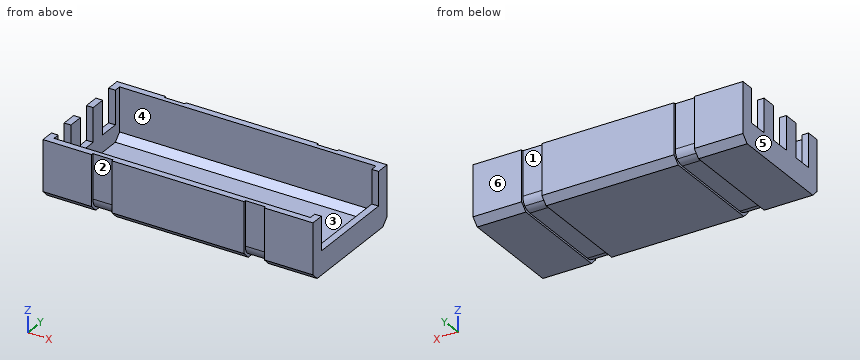
```python
from build123d import *

# Parameters (mm, degrees)
F0_W         = 40
F0_H         = 17.5
F1_DEPTH     = 8.5
F2_T         = -1
F3_W         = 1
F3_H         = 3
F4_DEPTH     = 5
F5_SIZE      = 1
F8_W         = 3
F8_H         = 1
F8_H_2       = 7.5
F11_DEPTH    = 0.3
F7_W         = 3
F7_H         = 1.4142135624
F12_DEPTH    = 0.3
F6_W         = 3
F6_H         = 15.5
F13_DEPTH    = 0.3
F9_W         = 3
F9_H         = 7.5
F14_DEPTH    = 0.3
F10_W        = 3
F10_H        = 5.3033008589
F10_H_2      = 1.4142135624
F15_DEPTH    = 0.3
F16_T1_DEPTH = 3
F16_T3_DEPTH = 3
F18_W        = 2.25
F18_H        = 5
F19_DEPTH    = 25


# Not quite as in the source:
# - a fillet or chamfer that OpenCascade refuses, or shapes differently, is made with other operations: its cross-section is extruded or revolved along the edge and cut away or added
# - two fillets or chamfers of one size are made in one step


with BuildPart() as f1:
    # F0 (on Top) → F1 (new body)
    with BuildSketch(Plane.XY):
        with Locations((-65.668810606, 16.5984117985)):
            Rectangle(F0_W, F0_H)
    extrude(amount=F1_DEPTH)

    # F2
    f2_openings = [f1.faces().sort_by_distance(p)[0] for p in [
        (-65.668811, 16.598412, 8.5),
    ]]
    offset(amount=F2_T, openings=f2_openings)

    # F3 (on face) → F4 (cut)
    with BuildSketch(Plane.XY.offset(8.5)):
        with Locations((-85.168810606, 21.8484117985)):
            Rectangle(F3_W, F3_H)
        with Locations((-85.168810606, 16.5984117985)):
            Rectangle(F3_W, F3_H)
        with Locations((-85.168810606, 11.3484117985)):
            Rectangle(F3_W, F3_H)
        with Locations((-46.168810606, 11.3484117985)):
            Rectangle(F3_W, F3_H)
        with Locations((-46.168810606, 16.5984117985)):
            Rectangle(F3_W, F3_H)
        with Locations((-46.168810606, 21.8484117985)):
            Rectangle(F3_W, F3_H)
    extrude(amount=-F4_DEPTH, mode=Mode.SUBTRACT)

    # F5
    f5_edges = [f1.edges().sort_by_distance(p)[0] for p in [
        (-65.668811, 7.848412, 0),
        (-65.668811, 25.348412, 0),
        (-65.668811, 24.348412, 1),
        (-65.668811, 8.848412, 1),
    ]]
    chamfer(f5_edges, length=F5_SIZE)

    # F8 (on face) → F11 (cut)
    with BuildSketch(Plane(origin=(0, 25.3484117985, 0), x_dir=(-1, 0, 0), z_dir=(0, 1, 0))):
        with Locations((76.9616991878, 0.5)):
            Rectangle(F8_W, F8_H)
        with Locations((76.9616991878, 4.75)):
            Rectangle(F8_W, F8_H_2)
        with Locations((54.3759220243, 4.75)):
            Rectangle(F8_W, F8_H_2)
    extrude(amount=-F11_DEPTH, mode=Mode.SUBTRACT)

    # F7 (on face) → F12 (cut)
    with BuildSketch(Plane(origin=(0, 12.1742058992, -12.1742058992), x_dir=(1, 0, 0), z_dir=(0, 0.7071067812, -0.7071067812))):
        with Locations((-76.9616991878, -17.924033875)):
            Rectangle(F7_W, F7_H)
        with Locations((-54.3759220243, -17.924033875)):
            Rectangle(F7_W, F7_H)
    extrude(amount=-F12_DEPTH, mode=Mode.SUBTRACT)

    # F6 (on face) → F13 (cut)
    with BuildSketch(Plane(origin=(0, 0, 0), x_dir=(1, 0, 0), z_dir=(0, 0, -1))):
        with Locations((-76.9616991878, -16.5984117985)):
            Rectangle(F6_W, F6_H)
        with Locations((-54.3759220243, -16.5984117985)):
            Rectangle(F6_W, F6_H)
    extrude(amount=-F13_DEPTH, mode=Mode.SUBTRACT)

    # F9 (on face) → F14 (cut)
    with BuildSketch(Plane.XZ.offset(-7.8484117985)):
        with Locations((-76.9616991878, 4.75)):
            Rectangle(F9_W, F9_H)
        with Locations((-54.3759220243, 4.75)):
            Rectangle(F9_W, F9_H)
    extrude(amount=-F14_DEPTH, mode=Mode.SUBTRACT)

    # F10 (on face) → F15 (cut)
    with BuildSketch(Plane(origin=(0, 4.4242058992, 4.4242058992), x_dir=(1, 0, 0), z_dir=(0, -0.7071067812, -0.7071067812))):
        with Locations((-76.9616991878, -2.1909079936)):
            Rectangle(F10_W, F10_H)
        with Locations((-76.9616991878, -5.5496652042)):
            Rectangle(F10_W, F10_H_2)
        with Locations((-54.3759220243, -5.5496652042)):
            Rectangle(F10_W, F10_H_2)
    extrude(amount=-F15_DEPTH, mode=Mode.SUBTRACT)

    # F16: fillet of radius 2 on 8 edges, made by hand

    # F16_s2 → F16_t1 (cut)
    with BuildSketch(Plane.YZ.offset(-55.8759220243)):
        with BuildLine():
            ThreePointArc((8.7341982361, 0.5384776311), (8.3006527335, 1.1873243287), (8.1484117985, 1.9526911935))
            Line((8.1484117985, 1.9526911935), (8.1484117985, 1.1242640687))
            Line((8.1484117985, 1.1242640687), (8.7341982361, 0.5384776311))
        make_face()
        with BuildLine():
            ThreePointArc((9.8011029919, 0.3), (9.0357361272, 0.452240935), (8.3868894296, 0.8857864376))
            Line((8.3868894296, 0.8857864376), (8.9726758672, 0.3))
            Line((8.9726758672, 0.3), (9.8011029919, 0.3))
        make_face()
        with BuildLine():
            ThreePointArc((25.0484117985, 1.9526911935), (24.8961708635, 1.1873243287), (24.4626253609, 0.5384776311))
            Line((24.4626253609, 0.5384776311), (25.0484117985, 1.1242640687))
            Line((25.0484117985, 1.1242640687), (25.0484117985, 1.9526911935))
        make_face()
        with BuildLine():
            ThreePointArc((24.8099341674, 0.8857864376), (24.1610874697, 0.452240935), (23.395720605, 0.3))
            Line((23.395720605, 0.3), (24.2241477298, 0.3))
            Line((24.2241477298, 0.3), (24.8099341674, 0.8857864376))
        make_face()
    extrude(amount=F16_T1_DEPTH, mode=Mode.SUBTRACT)

    # F16_s4 → F16_t3 (cut)
    with BuildSketch(Plane.YZ.offset(-78.4616991878)):
        with BuildLine():
            ThreePointArc((9.8011029919, 0.3), (9.0357361272, 0.452240935), (8.3868894296, 0.8857864376))
            Line((8.3868894296, 0.8857864376), (8.9726758672, 0.3))
            Line((8.9726758672, 0.3), (9.8011029919, 0.3))
        make_face()
        with BuildLine():
            ThreePointArc((8.7341982361, 0.5384776311), (8.3006527335, 1.1873243287), (8.1484117985, 1.9526911935))
            Line((8.1484117985, 1.9526911935), (8.1484117985, 1.1242640687))
            Line((8.1484117985, 1.1242640687), (8.7341982361, 0.5384776311))
        make_face()
        with BuildLine():
            ThreePointArc((24.8099341674, 0.8857864376), (24.1610874697, 0.452240935), (23.395720605, 0.3))
            Line((23.395720605, 0.3), (24.2241477298, 0.3))
            Line((24.2241477298, 0.3), (24.8099341674, 0.8857864376))
        make_face()
        with BuildLine():
            ThreePointArc((25.0484117985, 1.9526911935), (24.8961708635, 1.1873243287), (24.4626253609, 0.5384776311))
            Line((24.4626253609, 0.5384776311), (25.0484117985, 1.1242640687))
            Line((25.0484117985, 1.1242640687), (25.0484117985, 1.9526911935))
        make_face()
    extrude(amount=F16_T3_DEPTH, mode=Mode.SUBTRACT)

    # F18 (on face) → F19 (cut)
    with BuildSketch(Plane.YZ.offset(-45.668810606)):
        with Locations((13.9734117985, 6)):
            Rectangle(F18_W, F18_H)
        with Locations((19.2234117985, 6)):
            Rectangle(F18_W, F18_H)
    extrude(amount=-F19_DEPTH, mode=Mode.SUBTRACT)


solid = f1.part
```
Input: part model. Units: mm. Frame: model coordinates. Face numbers are marked on the shaded views. A direction names the side the tool comes from. Round coordinates to 2 decimals unless told otherwise and drop trailing zeros. Write each loop counter-clockwise with the first axis right and the second up, starting at its lowest first coordinate (ties: lowest second). Pieces come first, ordered by that corner, then holes. Notation, with made-up numbers: M 5,-30.75 L 14,-30.75 A13 ccw 14,-7.75 Z; hole C 40,-18 d4. An arc over 180 degrees is marked long. Write each question's results on one line, items separated by ' | '.
Q1. Pin query (flat end, axial travel): P1, Ø2.5, axis at y = 16.5, z = 6.5, coming from the -X side. Return the tip coordinate at first contact, or that it passes through.
Results:
P1: passes through
Q2. Section query C-C (z = 3). Return loops of the section in (x, y).
Results:
outline: M -85.67,7.85 L -78.46,7.85 L -78.46,8.15 L -75.46,8.15 L -75.46,7.85 L -55.88,7.85 L -55.88,8.15 L -52.88,8.15 L -52.88,7.85 L -45.67,7.85 L -45.67,25.35 L -52.88,25.35 L -52.88,25.05 L -55.88,25.05 L -55.88,25.35 L -75.46,25.35 L -75.46,25.05 L -78.46,25.05 L -78.46,25.35 L -85.67,25.35 Z; hole M -84.67,8.85 L -46.67,8.85 L -46.67,24.35 L -84.67,24.35 Z
Q3. Section query D-D (z = 7.5). State how many separate pieces and enclosed holes the cut face has, and give its area (3 significant figures).
Results:
separate pieces: 4 | enclosed holes: 0 | area: 84.9 mm^2
Q4. Draft query along Y for the marked faces 4, 5 and 6. Return one class per face: released by +Y, released by -Y, zero draft, split by the parting line, or undercut.
Results:
face 4: undercut | face 5: zero draft | face 6: released by +Y
Q5. Section query A-A (y = 10.25). Return loops of the section in (x, z), and give its area (3 significant figures).
Results:
outline: M -85.67,0 L -78.46,0 L -78.46,0.3 L -75.46,0.3 L -75.46,0 L -55.88,0 L -55.88,0.3 L -52.88,0.3 L -52.88,0 L -45.67,0 L -45.67,3.5 L -46.67,3.5 L -46.67,1 L -84.67,1 L -84.67,3.5 L -85.67,3.5 Z | area: 43.2 mm^2
Q6. Line query: line 1 along Y through (x, z) = (-74.5, 6); line 2 along X through (y, z) = (19.5, 2.75); line 3 along X through (y, z) = (13.75, 6). Output: solid intervals per line, ascending.
Results:
line 1: y = 7.85 to 8.85, 24.35 to 25.35 | line 2: x = -85.67 to -84.67, -46.67 to -45.67 | line 3: x = -85.67 to -84.67
Q7. Section query B-B (x = -79.5). Return loops of the section in (y, z), and give its area (3 significant figures).
Results:
outline: M 7.85,1 L 8.85,0 L 24.35,0 L 25.35,1 L 25.35,8.5 L 24.35,8.5 L 24.35,2 L 23.35,1 L 9.85,1 L 8.85,2 L 8.85,8.5 L 7.85,8.5 Z | area: 32.5 mm^2
Q8. Access query for the marked faces 1, 2 and 3. Directions: +Z, -Z, +X, -X, +Y, -Y. A direction counts if a zero-diameter tool reaches every point of the face in a straight line with its end or side. Return the directions, or none.
Results:
face 1: +Z, -Z, +Y | face 2: +Z, -Z, -Y | face 3: +Z
